```python
from build123d import *

# Parameters (mm, degrees)
F0_W     = 2.54
F0_H     = 17.145
F0_W_2   = 3.175
F0_H_2   = 2.54
F0_H_3   = 3.175
F0_W_3   = 17.145
F1_DEPTH = 2.54
F2_DEPTH = 24.765
F3_DEPTH = 38.1


with BuildPart() as f1:
    # F0 (on Top) → F1 (new body)
    with BuildSketch(Plane.XY):
        with Locations((1.27, 16.8275)):
            Rectangle(F0_W, F0_H)
        with Locations((4.1275, 16.8275)):
            Rectangle(F0_W_2, F0_H)
        with Locations((6.985, 16.8275)):
            Rectangle(F0_W, F0_H)
        with Locations((1.27, 6.985)):
            Rectangle(F0_W, F0_H_2)
        with Locations((1.27, 4.1275)):
            Rectangle(F0_W, F0_H_3)
        with Locations((1.27, 1.27)):
            Rectangle(F0_W, F0_H_2)
        with Locations((4.1275, 1.27)):
            Rectangle(F0_W_2, F0_H_2)
        with Locations((4.1275, 4.1275)):
            Rectangle(F0_W_2, F0_H_3)
        with Locations((4.1275, 6.985)):
            Rectangle(F0_W_2, F0_H_2)
        with Locations((6.985, 4.1275)):
            Rectangle(F0_W, F0_H_3)
        with Locations((6.985, 6.985)):
            Rectangle(F0_W, F0_H_2)
        with Locations((6.985, 1.27)):
            Rectangle(F0_W, F0_H_2)
        with Locations((16.8275, 1.27)):
            Rectangle(F0_W_3, F0_H_2)
        with Locations((16.8275, 4.1275)):
            Rectangle(F0_W_3, F0_H_3)
        with Locations((16.8275, 6.985)):
            Rectangle(F0_W_3, F0_H_2)
    extrude(amount=F1_DEPTH)

    # F0 (on Top) → F2 (join)
    with BuildSketch(Plane.XY):
        with Locations((6.985, 16.8275)):
            Rectangle(F0_W, F0_H)
        with Locations((6.985, 6.985)):
            Rectangle(F0_W, F0_H_2)
        with Locations((16.8275, 6.985)):
            Rectangle(F0_W_3, F0_H_2)
    extrude(amount=F2_DEPTH)

    # F0 (on Top) → F3 (join)
    with BuildSketch(Plane.XY):
        with Locations((1.27, 16.8275)):
            Rectangle(F0_W, F0_H)
        with Locations((1.27, 6.985)):
            Rectangle(F0_W, F0_H_2)
        with Locations((1.27, 4.1275)):
            Rectangle(F0_W, F0_H_3)
        with Locations((1.27, 1.27)):
            Rectangle(F0_W, F0_H_2)
        with Locations((4.1275, 1.27)):
            Rectangle(F0_W_2, F0_H_2)
        with Locations((6.985, 1.27)):
            Rectangle(F0_W, F0_H_2)
        with Locations((16.8275, 1.27)):
            Rectangle(F0_W_3, F0_H_2)
    extrude(amount=F3_DEPTH)


solid = f1.part
```
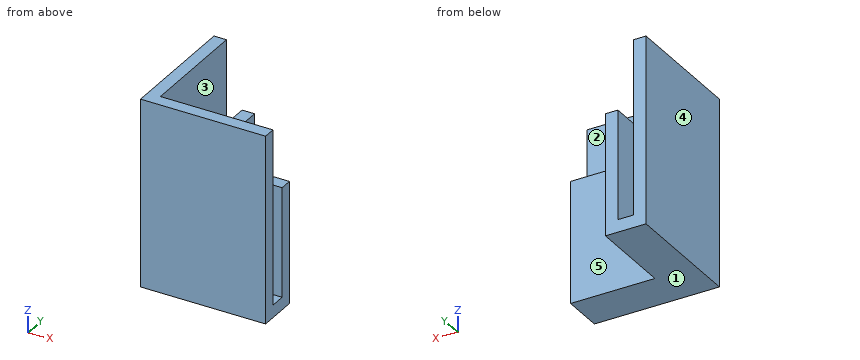
Input: part model. Units: mm. Frame: model coordinates. Face numbers are marked on the shaded views. A direction names the side the tool comes from. Coordinates: 2 decimals unless noted, no trailing zeros. Write each loop counter-clockwise with the first axis right and the second up, starting at its lowest first coordinate (ties: lowest second). Pieces come first, ordered by that corner, then holes. Notation, with made-up numbers: (42, 27.25) - (60, 27.25) arc R19 cw to (60, 58.25) - close; hole circle Ø10 at (-14.5, -12). An arc over 180 degrees is marked (long way). Put each result on its own line as item: value. Start each with the question number.
1) Cut plane D-D (z = 28). Return the cut outline in (x, y).
2) Contact query for flat-ended pins moving along their axis: pin 1 (6 mm diameter, centred on x = 22.5, y = 11, fed in from +Z) (3 decimals); pin 2 (4 mm diameter, centred on y = 20, z = 27.5, fed in from +X); pin 3 (8 mm diameter, centred on y = 20.5, z = 4, fed in from +X) (3 decimals). Output: stop coordinate, or through.
3) Cut plane A-A (z = 18). Return the cut outline in (x, y) (3 decimals).
4) Cut plane B-B (x = 10.5). Return the cut outline in (y, z) (3 decimals), plus the area to 3 significant figures.
5) Mould query, pull axis X, two halves, no side actions, for the marked faces 3, 4 and 5. Classes: pulls with the +X half, pulls with the -X half, needs draft (parallel to the pull), parting line crosses it, or undercut.
6) Ray query, L1, parallel to Y at x = 19.75, z = 10 (3 decimals); L2, parallel to X at y = 10.5, z = 26.5. Return the intervals inside material, ascending.
7) Reachability of the marked faces 1 and 2 from +Z, -Z, +X, -X, +Y, -Y: full face, straight path, thin tool, end or side. Return the list, or none.
Resolved:
1. outline: (0, 0) - (25.4, 0) - (25.4, 2.54) - (2.54, 2.54) - (2.54, 25.4) - (0, 25.4) - close
2. pin 1: stops at z = 24.765
2. pin 2: stops at x = 2.54
2. pin 3: stops at x = 8.255
3. outline: (0, 0) - (25.4, 0) - (25.4, 2.54) - (2.54, 2.54) - (2.54, 25.4) - (0, 25.4) - close; (5.715, 5.715) - (25.4, 5.715) - (25.4, 8.255) - (8.255, 8.255) - (8.255, 25.4) - (5.715, 25.4) - close
4. outline: (0, 0) - (8.255, 0) - (8.255, 24.765) - (5.715, 24.765) - (5.715, 2.54) - (2.54, 2.54) - (2.54, 38.1) - (0, 38.1) - close
4. area: 168 mm2
5. face 3: undercut
5. face 4: pulls with the -X half
5. face 5: needs draft
6. L1: y = 0 to 2.54, 5.715 to 8.255
6. L2: x = 0 to 2.54
7. face 1: -Z, +X, -X, +Y, -Y
7. face 2: +Z, +X
